CAD build for the part. Positions are in the model's coordinates, mm. A direction names the side the tool comes from. Coordinates: 2 decimals unless noted, no trailing zeros. Order: outer loops, then holes, each group sorted by start corner. A loop starts at its lowest first (then second) coordinate and runs counter-clockwise, first axis right, second up. Notation, with made-up numbers: M 49.25,8.25 L 108.25,8.25 A22 cw 108.25,38.25 Z; hole C 21.25,76.25 d7. An arc over 180 degrees is marked long. One line per item, written item: value.
from build123d import *

# Parameters (mm, degrees)
SKETCH1_W             = 60
SKETCH1_H             = 18
BOSS_EXTRUDE1_DEPTH   = 26
SKETCH2_R             = 3.85
EYESHAFT_HOLES_DEPTH  = 15
EYESHAFT_FILLET_R     = 3
SKETCH5_W             = 5
SKETCH5_H             = 2.2
FRONT_LEG_HOLES_DEPTH = 13
SKETCH7_W             = 10.2
SKETCH7_H             = 3.3
BACK_LEGS_DEPTH       = 13
SKETCH18_W            = 15.65
SKETCH18_H            = 35.9
BOSS_EXTRUDE2_DEPTH   = 26
SKETCH19_W            = 11.75
SKETCH19_H            = 31.9
CUT_EXTRUDE9_DEPTH    = 9.35
SKETCH20_W            = 11.75
SKETCH20_H            = 23.9
CUT_EXTRUDE10_DEPTH   = 15
FILLET4_R             = 2
CHAMFER1_SIZE         = 1
SKETCH21_W            = 9
SKETCH21_H            = 4
CUT_EXTRUDE11_DEPTH   = 15
FILLET5_R             = 2
SKETCH22_R            = 0.75
CUT_EXTRUDE12_DEPTH   = 3


with BuildPart() as part:
    # Sketch1 → Boss-Extrude1 (new body)
    with BuildSketch(Plane(origin=(0, 0, 0), x_dir=(1, 0, 0), z_dir=(0, 1, 0))):
        Rectangle(SKETCH1_W, SKETCH1_H)
    extrude(amount=BOSS_EXTRUDE1_DEPTH)

    # Sketch2 → Eyeshaft holes (cut)
    with BuildSketch(Plane(origin=(0, 26, 0), x_dir=(1, 0, 0), z_dir=(0, 1, 0))):
        with Locations(Location((-22, -3, 0), (0, 0, 270))):
            Circle(SKETCH2_R)
        with Locations(Location((22, -3, 0), (0, 0, 270))):
            Circle(SKETCH2_R)
    extrude(amount=-EYESHAFT_HOLES_DEPTH, mode=Mode.SUBTRACT)

    # Eyeshaft Fillet
    eyeshaft_fillet_edges = [part.edges().sort_by_distance(p)[0] for p in [
        (-22, 11, -0.85),
        (22, 11, -0.85),
    ]]
    fillet(eyeshaft_fillet_edges, radius=EYESHAFT_FILLET_R)

    # Sketch5 → Front leg holes (cut)
    with BuildSketch(Plane(origin=(0, 26, 0), x_dir=(1, 0, 0), z_dir=(0, 1, 0))):
        with Locations((-12, -3)):
            Rectangle(SKETCH5_W, SKETCH5_H)
        with Locations((12, -3)):
            Rectangle(SKETCH5_W, SKETCH5_H)
    extrude(amount=-FRONT_LEG_HOLES_DEPTH, mode=Mode.SUBTRACT)

    # Sketch7 → Back Legs (cut)
    with BuildSketch(Plane(origin=(0, 26, 0), x_dir=(1, 0, 0), z_dir=(0, 1, 0))):
        with Locations((-13.9, 5.4)):
            Rectangle(SKETCH7_W, SKETCH7_H)
        with Locations((13.9, 5.4)):
            Rectangle(SKETCH7_W, SKETCH7_H)
    extrude(amount=-BACK_LEGS_DEPTH, mode=Mode.SUBTRACT)

    # Sketch18 → Boss-Extrude2 (add)
    with BuildSketch(Plane(origin=(0, 26, 0), x_dir=(1, 0, 0), z_dir=(0, 1, 0))):
        with Locations((0, 3.1)):
            Rectangle(SKETCH18_W, SKETCH18_H)
    extrude(amount=-BOSS_EXTRUDE2_DEPTH)

    # Sketch19 → Cut-Extrude9 (cut)
    with BuildSketch(Plane(origin=(0, 26, 0), x_dir=(1, 0, 0), z_dir=(0, 1, 0))):
        with Locations((0, 3.1)):
            Rectangle(SKETCH19_W, SKETCH19_H)
    extrude(amount=-CUT_EXTRUDE9_DEPTH, mode=Mode.SUBTRACT)

    # Sketch20 → Cut-Extrude10 (cut)
    with BuildSketch(Plane(origin=(0, 16.65, 0), x_dir=(1, 0, 0), z_dir=(0, 1, 0))):
        with Locations((0, 3.1)):
            Rectangle(SKETCH20_W, SKETCH20_H)
    extrude(amount=-CUT_EXTRUDE10_DEPTH, mode=Mode.SUBTRACT)

    # Fillet4
    fillet4_edges = [part.edges().sort_by_distance(p)[0] for p in [
        (30, 13, 9),
        (-30, 13, 9),
        (-30, 13, -9),
        (30, 13, -9),
        (-7.825, 13, 14.85),
        (7.825, 13, -21.05),
        (-7.825, 13, -21.05),
        (-7.825, 13, -9),
        (-7.825, 13, 9),
        (7.825, 13, 14.85),
        (7.825, 13, -9),
        (7.825, 13, 9),
    ]]
    fillet(fillet4_edges, radius=FILLET4_R)

    # Chamfer1
    chamfer1_edges = [part.edges().sort_by_distance(p)[0] for p in [
        (-22, 26, -0.85),
        (22, 26, -0.85),
        (-9.5, 26, 3),
        (-12, 26, 1.9),
        (-14.5, 26, 3),
        (-12, 26, 4.1),
        (14.5, 26, 3),
        (12, 26, 1.9),
        (9.5, 26, 3),
        (12, 26, 4.1),
        (-19, 26, -5.4),
        (-13.9, 26, -3.75),
        (-8.8, 26, -5.4),
        (-13.9, 26, -7.05),
        (8.8, 26, -5.4),
        (13.9, 26, -3.75),
        (19, 26, -5.4),
        (13.9, 26, -7.05),
    ]]
    chamfer(chamfer1_edges, length=CHAMFER1_SIZE)

    # Sketch21 → Cut-Extrude11 (cut)
    with BuildSketch(Plane(origin=(0, 0, 8.85), x_dir=(-1, 0, 0), z_dir=(0, 0, -1))):
        with Locations((0, 3.65)):
            Rectangle(SKETCH21_W, SKETCH21_H)
    extrude(amount=-CUT_EXTRUDE11_DEPTH, mode=Mode.SUBTRACT)

    # Fillet5
    fillet5_edges = [part.edges().sort_by_distance(p)[0] for p in [
        (0, 5.65, 8.85),
    ]]
    fillet(fillet5_edges, radius=FILLET5_R)

    # Sketch22 → Cut-Extrude12 (cut)
    with BuildSketch(Plane(origin=(0, 16.65, 0), x_dir=(1, 0, 0), z_dir=(0, 1, 0))):
        with Locations(Location((0, 17.3, 0), (0, 0, 270))):
            Circle(SKETCH22_R)
        with Locations(Location((0, -11.1, 0), (0, 0, 270))):
            Circle(SKETCH22_R)
    extrude(amount=-CUT_EXTRUDE12_DEPTH, mode=Mode.SUBTRACT)


solid = part.part
Q1. Slice it at D-D (z = -17.3). List the corners of the cut face in (x, y) (3 decimals), plus the area to 3 significant figures.
Recorded:
outline: M -7.825,0 L 7.825,0 L 7.825,26 L 5.875,26 L 5.875,16.65 L 0.75,16.65 L 0.75,13.65 L -0.75,13.65 L -0.75,16.65 L -5.875,16.65 L -5.875,26 L -7.825,26 Z
area: 293 mm^2
Q2. Slice it at C-C (y = 20). Give the number of separate pieces and of enclosed holes in the cut face, plus the area to 3 significant figures.
Recorded:
separate pieces: 1
enclosed holes: 7
area: 799 mm^2
Q3. Which spindle directions (+Z, -Z, +X, -X, +Y, -Y) get a long thin tool onto all of the face, cutting with end or side? Do faces 4 (the face through (-7.3, 12.8, -20.4)), 5 (the face through (0, 1.65, 0)), 6 (the face through (-9.5, 19, 3)), 7 (the face through (29.4, 13.18, 8.43)), 8 (the face through (0, 5.65, 13)). Say none if no direction does.
Recorded:
face 4: -Z, -X, +Y, -Y
face 5: none
face 6: +Y
face 7: +Z, +X, +Y, -Y
face 8: +Z
Q4. Slice it at A-A (x = -1.5). List the corners of the cut face in (y, z), plus the area to 3 significant figures.
Recorded:
outline: M 0,-21.05 L 26,-21.05 L 26,-19.05 L 16.65,-19.05 L 16.65,-15.05 L 1.65,-15.05 L 1.65,14.85 L 0,14.85 Z; M 5.65,10.85 A2 ccw 7.65,8.85 L 16.65,8.85 L 16.65,12.85 L 26,12.85 L 26,14.85 L 5.65,14.85 Z
area: 252 mm^2
Q5. Mould opens along Z. For faces 1 (the face through (-7.825, 13, 12)), 2 (the face through (0.03, 15.17, 10.35)), 3 (the face through (19, 13, 9)) say: released by +Z, released by -Z, zero draft, split by the parting line, or undercut.
Recorded:
face 1: zero draft
face 2: undercut
face 3: released by +Z
Q6. Pin check, flat tips, straight feed: pin 1 Ø14.5 at (x, y) = (-22, 11.5) entering from -Z; pin 2 Ø5.5 at (x, y) = (13, 21.5) entering from +Z; pin 3 Ø1.4 at (x, z) = (22, 3) entering from +Y. Stop position of each tip, or through.
Recorded:
pin 1: stops at z = -9
pin 2: stops at z = 9
pin 3: stops at y = 11
Q7. Slice it at B-B (z = -12). List the corners of the cut face in (x, y) (3 decimals).
Recorded:
outline: M -7.825,0 L 7.825,0 L 7.825,26 L 5.875,26 L 5.875,1.65 L -5.875,1.65 L -5.875,26 L -7.825,26 Z
Q8. Drill centre lines: line 1 along X through (y, z) = (20, 3) (3 decimals); line 2 along Z through (x, y) = (10.5, 19.5). Where is each one in solid material? Low to high.
Recorded:
line 1: x = -30 to -25.85, -18.15 to -14.5, -9.5 to -5.875, 5.875 to 9.5, 14.5 to 18.15, 25.85 to 30
line 2: z = -9 to -7.05, -3.75 to 1.9, 4.1 to 9
